Autodesk Inventor part; units mm, degrees
ref_plane "YZ Plane" through (0, 0, 0) normal (1, 0, 0) x (0, 1, 0)
ref_plane "XZ Plane" through (0, 0, 0) normal (0, 1, 0) x (-1, 0, 0)
ref_plane "XY Plane" through (0, 0, 0) normal (0, 0, 1) x (1, 0, 0)
sketch "Sketch1" plane through (0, 0, 0) normal (0, 0, 1) x (1, 0, 0)
  circle A0 centre (0, 0) radius 215.9
  line L0 (-215.9, 215.9) -> (215.9, 215.9)
  line L1 (215.9, 215.9) -> (215.9, -215.9)
  line L2 (215.9, -215.9) -> (-215.9, -215.9)
  line L3 (-215.9, -215.9) -> (-215.9, 215.9)
  point P0 (215.9, 0)
  point P1 (0, 215.9)
  dimension "d0" = 431.8
  dimension "d1" = 431.8
  dimension "d2" = 431.8
  dimension "d3" = 215.9
  dimension "d4" = 215.9
extrude "Extrusion1" add sketch "Sketch1" along normal blind 11.938 contours A0 L0 L1
sketch "Sketch2" plane through (0, 0, 11.938) normal (0, 0, 1) x (1, 0, 0)
  circle A0 centre (0, 0) radius 220
  dimension "d7" = 440
extrude "Extrusion2" cut sketch "Sketch2" against normal through all
sketch "Sketch3" plane through (0, 0, 11.938) normal (0, 0, 1) x (1, 0, 0)
  line L0 (215.9, 215.9) -> (42.2752, 215.9)
  line L1 (215.9, 215.9) -> (197.9422, 215.9)
  line L2 (215.9, 42.2752) -> (215.9, 215.9)
  line L3 (215.9, 215.9) -> (215.9, 197.9368)
  line L4 (215.9, 197.9368) -> (135.0791, 117.1158)
  line L5 (135.0791, 117.1158) -> (117.1185, 135.0763)
  line L6 (117.1185, 135.0763) -> (197.9422, 215.9)
  point P0 (0, 0)
  dimension "d10" = 25.4
  dimension "d11" = 135
  dimension "d12" = 135
  dimension "d13" = 17.9578
  dimension "d14" = 90
  dimension "d15" = 127
extrude "Extrusion3" cut sketch "Sketch3" against normal blind 8.89
sketch "Sketch5" plane through (0, 0, 11.938) normal (0, 0, 1) x (1, 0, 0)
  arc A0 (164.2856, 146.3224) -> (146.3253, 164.2831) centre (0, 0) ccw
  line L0 (215.9, 197.9368) -> (164.2856, 146.3224)
  line L1 (215.9, 215.9) -> (215.9, 197.9368)
  line L2 (197.9422, 215.9) -> (215.9, 215.9)
  line L3 (146.3253, 164.2831) -> (197.9422, 215.9)
  line L4 (137.2766, 157.4974) -> (211.5205, 231.7413)
  line L5 (211.5205, 231.7413) -> (233.2717, 213.0454)
  line L6 (233.2717, 213.0454) -> (157.5001, 137.2738)
  line L7 (157.5001, 137.2738) -> (137.2766, 157.4974)
  dimension "d22" = 90
  dimension "d25" = 4.32
  dimension "d26" = 1.6002
  dimension "d27" = 1.6002
extrude "Extrusion5" cut sketch "Sketch5" against normal up to surface (8.89 mm away) contours A0 L3 L2 L1 L0 | L4 L5 L6 L7
properties part number "Wind Tunnel Fan Shroud Corner Mod Strap" material "Wood (Oak)"
Design review of the part built by this model. Coordinates are the model's own, in mm. A direction names the side the tool comes from. Round coordinates to 2 decimals unless told otherwise and drop trailing zeros. Write each loop counter-clockwise with the first axis right and the second up, starting at its lowest first coordinate (ties: lowest second). Pieces come first, ordered by that corner, then holes. Notation, with made-up numbers: (0, 3.5) -> (9, 3.5) arc R23 cw to (9, 20.5) -> close; hole circle Ø1 at (-33, 38.5). An arc over 180 degrees is marked (long way). Answer in a Markdown table with one row per item.
Q1. Take a section at C-C, the plane y = 172. State the section outline as (x, z) points.
The answers:
| item | result |
|---|---|
| outline | (137.17, 0) -> (215.9, 0) -> (215.9, 11.94) -> (192.23, 11.94) -> (192.23, 3.05) -> (151.78, 3.05) -> (151.78, 11.94) -> (137.17, 11.94) -> close |
Q2. Clearance check with flat-ended pins moving along their axes: pin 1 Ø6 at (y, z) = (187.5, 8) entering from -X; pin 2 Ø5 at (y, z) = (184.5, 8) entering from -X; pin 3 Ø6 at (y, z) = (92.5, 5.5) entering from -X. State where each tip first meets the part, or that it passes through.
The answers:
| item | result |
|---|---|
| pin 1 | x = 110.04 |
| pin 2 | x = 115.89 |
| pin 3 | x = 198.19 |
Q3. Take a section at A-A, the plane z = 6.5. State the section outline as (x, y) points (3 decimals), then the cut area to 3 significant figures.
The answers:
| item | result |
|---|---|
| outline | (42.275, 215.9) arc R220 cw to (145.124, 165.345) -> (195.679, 215.9) -> close; (165.348, 145.121) arc R220 cw to (215.9, 42.275) -> (215.9, 195.674) -> close |
| area | 6,590 mm² |
Q4. Take a section at D-D, the plane y = 115. State the section outline as (x, z) points.
The answers:
| item | result |
|---|---|
| outline | (187.55, 0) -> (215.9, 0) -> (215.9, 11.94) -> (187.55, 11.94) -> close |
Q5. Draft analysis for pull direction X (two halves, no side actions). For faces 1 (the face through (215.9, 130, 6)), 2 (the face through (202, 137, 11.938)), 3 (the face through (180, 181, 3.048)), 4 (the face through (156.848, 154.269, 2.073)), state which applies: +X half, -X half, draft (parallel to the pull), parting line (faces both ways), or undercut.
The answers:
| item | result |
|---|---|
| face 1 | +X half |
| face 2 | draft |
| face 3 | undercut |
| face 4 | -X half |
Q6. For faces 5 (the face through (170.05, 190.27, 7.56)), 6 (the face through (135, 202, 11.938)), list the 3-axis set-ups (+Z, -Z, +X, -X, +Y, -Y) from which the entire face can be reached by the end or side of a thin tool; tool diameter is ignored.
The answers:
| item | result |
|---|---|
| face 5 | +Z |
| face 6 | +Z, +X, -X, +Y, -Y |
Q7. Take a section at B-B, the plane x = 176. State the section outline as (y, z) points.
The answers:
| item | result |
|---|---|
| outline | (132, 0) -> (215.9, 0) -> (215.9, 11.94) -> (196.22, 11.94) -> (196.22, 3.05) -> (155.77, 3.05) -> (155.77, 11.94) -> (132, 11.94) -> close |
Q8. To check wall thickness, follow L1, parallel to X at y = 166.5, z = 11; L2, parallel to Z at x = 157.5, y = 167.5; L3, parallel to Y at x = 195, z = 3.5. State the ranges of each line that lie inside material, in increasing order. Write a range as [from, to].
The answers:
| item | result |
|---|---|
| L1 | [143.8, 146.28], [186.73, 215.9] |
| L2 | [0, 3.05] |
| L3 | [101.86, 174.77], [215.22, 215.9] |
